Source: CAD feature listing. Evaluate the final solid. Frame: model axes, mm. Coordinates: 2 decimals unless noted, no trailing zeros. Order: outer loops, then holes, each group sorted by start corner. A loop starts at its lowest first (then second) coordinate and runs counter-clockwise, first axis right, second up.
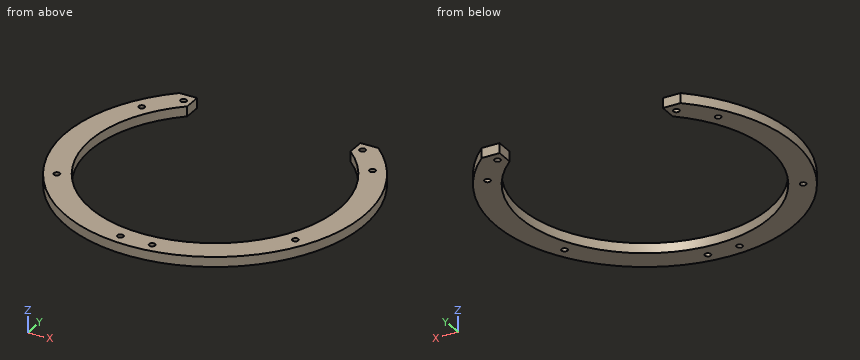
```python
from build123d import *

# Parameters (mm, degrees)
RESSALTO_EXTRUS_O1_DEPTH = 5
ESBO_O2_R                = 1.5
CORTE_EXTRUS_O1_DEPTH    = 311.009274327
ESBO_O3_W                = 82
ESBO_O3_H                = 18.792940288
CORTE_EXTRUS_O2_DEPTH    = 10


with BuildPart() as part:
    # Esboço1 → Ressalto-extrusão1 (new body)
    with BuildSketch(Plane.XY):
        with BuildLine():
            Line((44.495405461, -168.430491325), (22.44625518, -168.430491325))
            ThreePointArc((22.44625518, -168.430491325), (-5.504594539, -286.832190763), (-33.455444258, -168.430491325))
            Line((-33.455444258, -168.430491325), (-55.504594539, -168.430491325))
            ThreePointArc((-55.504594539, -168.430491325), (-5.504594539, -299.332190763), (44.495405461, -168.430491325))
        make_face()
    extrude(amount=RESSALTO_EXTRUS_O1_DEPTH)

    # Esboço2 → Corte-extrusão1 (cut, through all)
    with BuildSketch(Plane.XY.offset(5)):
        with Locations((39.44625518, -173.430491325)):
            Circle(ESBO_O2_R)
        with Locations((52.44625518, -187.430491325)):
            Circle(ESBO_O2_R)
        with Locations((54.44625518, -258.430491325)):
            Circle(ESBO_O2_R)
        with Locations(Location((-13.455444258, -293.430491325, 0), (0, 0, 180))):
            Circle(ESBO_O2_R)
        with Locations((2.44625518, -293.430491325)):
            Circle(ESBO_O2_R)
        with Locations(Location((-65.455444258, -258.430491325, 0), (0, 0, 180))):
            Circle(ESBO_O2_R)
        with Locations(Location((-63.455444258, -187.430491325, 0), (0, 0, 180))):
            Circle(ESBO_O2_R)
        with Locations(Location((-50.455444258, -173.430491325, 0), (0, 0, 180))):
            Circle(ESBO_O2_R)
    extrude(amount=-CORTE_EXTRUS_O1_DEPTH, mode=Mode.SUBTRACT)

    # Esboço3 → Corte-extrusão2 (cut)
    with BuildSketch(Plane.XY.offset(5)):
        with Locations((-5.504594539, -170.544921833)):
            Rectangle(ESBO_O3_W, ESBO_O3_H)
    extrude(amount=-CORTE_EXTRUS_O2_DEPTH, mode=Mode.SUBTRACT)


solid = part.part
```
1. Material intervals for line 1 along X through (y, z) = (-205, 1.6); line 2 along X through (y, z) = (-188.5, 3); line 3 along X through (y, z) = (-210, 2.25), sorted ascending.
2. Section query B-B, the plane z = 4.2. Count the separate pieces of the cut face and the enclosed holes in it, plus the area to 3 significant figures.
3. Contact query for flat-ended pins moving along their axis: P1, Ø5, axis at x = 54.45, y = -258.43, coming from the -Z side; P2, Ø1.5, axis at x = 17, z = 1.5, coming from the +Y side; P3, Ø2.5, axis at x = -50.46, y = -173.43, coming from the +Z side. Output: stop coordinate, or through.
4. Section query A-A, the plane y = -254. Output: boundary loops of the cut face in (x, z).
5. Section query D-D, the plane x = -5.5. Output: boundary loops of the cut face in (y, z), plus the area to 3 significant figures.
6. Section query C-C, the plane y = -191.5. Output: boundary loops of the cut face in (x, z).
Answer key:
1. line 1: x = -77.97 to -64.94, 53.93 to 66.96
1. line 2: x = -71.39 to -64.51, -62.4 to -56.71, 45.7 to 51.39, 53.5 to 60.38
1. line 3: x = -79.12 to -66.34, 55.33 to 68.11
2. separate pieces: 1
2. enclosed holes: 8
2. area: 4,180 mm2
3. P1: stops at z = 0
3. P2: stops at y = -282.34
3. P3: passes through
4. outline: (-74.39, 0) - (-60.51, 0) - (-60.51, 5) - (-74.39, 5) - close; (49.51, 0) - (63.38, 0) - (63.38, 5) - (49.51, 5) - close
5. outline: (-299.33, 0) - (-286.83, 0) - (-286.83, 5) - (-299.33, 5) - close
5. area: 62.5 mm2
6. outline: (-72.94, 0) - (-58.69, 0) - (-58.69, 5) - (-72.94, 5) - close; (47.68, 0) - (61.93, 0) - (61.93, 5) - (47.68, 5) - close
